Part print with two shaded views. Sizes in mm from the minimum x, y, z corner. A direction names the side the tool comes from. Round coordinates to 2 decimals unless told otherwise and drop trailing zeros. Order: outer loops, then holes, each group sorted by start corner. A loop starts at its lowest first (then second) coordinate and runs counter-clockwise, first axis right, second up. Notation, with made-up numbers: (14, 47) -> (44, 47) arc R13 ccw to (44, 67) -> close; hole circle Ø6 at (-22.5, -37). An arc over 180 degrees is marked (long way). Put each result on its own line as item: value. Start each with the question number.
Q1. 3-axis set-ups, long thin cutter, end or side, ignore diameter. For the marked faces 5, 6 and 7: which of +Z, -Z, +X, -X, +Y, -Y reach the whole face in a straight line?
Q2. Pull direction Z, two halves, no side cores. Call the marked faces 1, 2, 3 and 4: released by +Z, released by -Z, zero draft, split by the parting line, or undercut.
Q3. Cut at D-D, the plane z = 11.75. List the corners of the cut face in (x, y), and give its area (3 significant figures).
Q4. Cut at B-B, the plane z = 7.5. List the corners of the cut face in (x, y).
Q5. Cut at C-C, the plane y = 5.75. List the corners of the cut face in (x, z).
Q6. Cut at A-A, the plane x = 7. List the corners of the cut face in (y, z) (1 decimal).
Q7. Probe L1, parallel to Z at x = 7, y = 3; L2, parallel to Z at x = 10.25, y = 6; L3, parallel to Y at x = 13.25, z = 2.75. List the from-to ranges inside material, lowest first.
Q8. Flat gauge pins, fed straight in: P1, Ø0.8, axis at x = 8, z = 13, coming from the +Y side; P2, Ø1.5, axis at y = 2, z = 4.5, coming from the -X side; P3, Ø4.5, axis at x = 7, z = 7.5, coming from the +Y side. Where does each tip first touch, or does it go through?
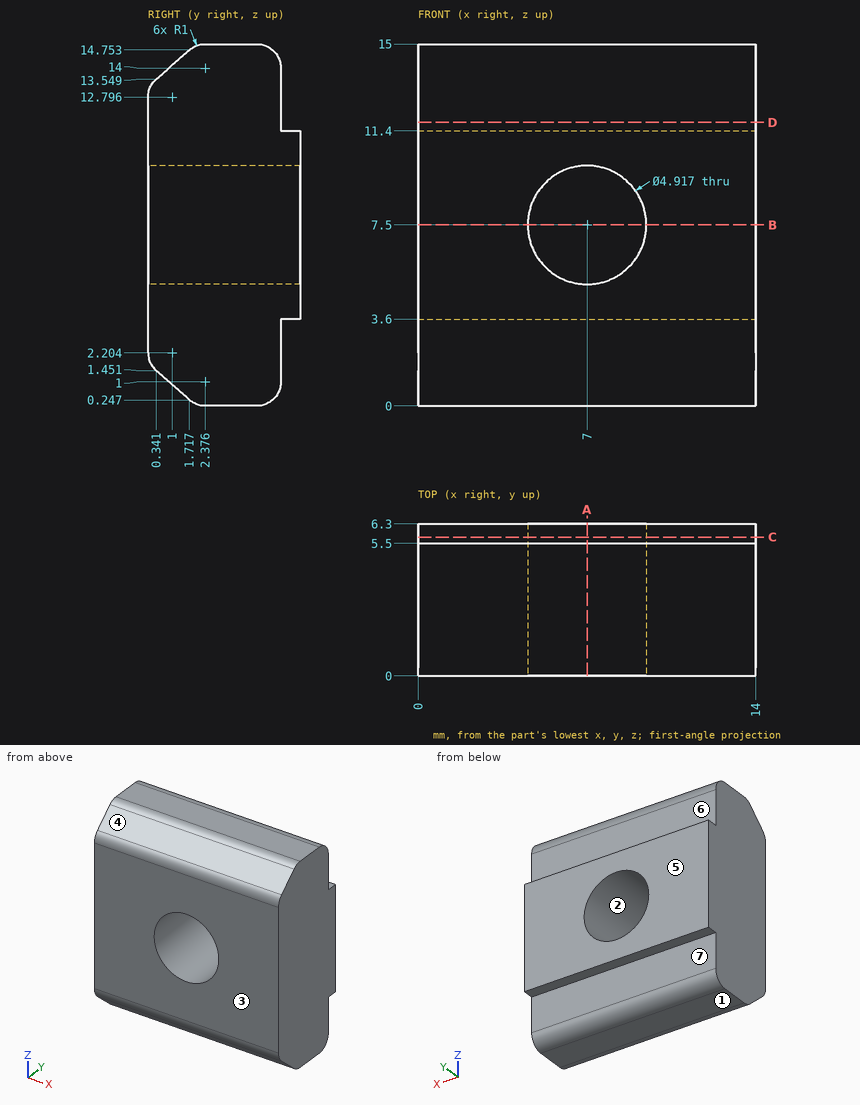
Ans:
1. face 5: +Z, -Z, +X, -X, +Y
1. face 6: +Z, +X, -X, +Y
1. face 7: -Z, +X, -X, +Y
2. face 1: released by -Z
2. face 2: undercut
2. face 3: zero draft
2. face 4: released by +Z
3. outline: (0, 0) -> (14, 0) -> (14, 5.5) -> (0, 5.5) -> close
3. area: 77.0 mm^2
4. outline: (0, 0) -> (4.54, 0) -> (4.54, 6.3) -> (0, 6.3) -> close; (9.46, 0) -> (14, 0) -> (14, 6.3) -> (9.46, 6.3) -> close
5. outline: (0, 3.6) -> (14, 3.6) -> (14, 11.4) -> (0, 11.4) -> close; hole circle Ø4.92 at (7, 7.5)
6. outline: (0, 2.2) arc R1 ccw to (0.3, 1.5) -> (1.7, 0.2) arc R1 ccw to (2.4, 0) -> (4.5, 0) arc R1 ccw to (5.5, 1) -> (5.5, 3.6) -> (6.3, 3.6) -> (6.3, 5) -> (0, 5) -> close; (0, 10) -> (6.3, 10) -> (6.3, 11.4) -> (5.5, 11.4) -> (5.5, 14) arc R1 ccw to (4.5, 15) -> (2.4, 15) arc R1 ccw to (1.7, 14.8) -> (0.3, 13.5) arc R1 ccw to (0, 12.8) -> close
7. L1: z = 0 to 5.04, 9.96 to 15
7. L2: z = 3.6 to 11.4
7. L3: y = 0 to 5.5
8. P1: stops at y = 5.5
8. P2: stops at x = 0
8. P3: passes through
